Could you check a few things on this model? Use its own coordinates, in mm. Coordinates: 2 decimals unless noted, no trailing zeros. Write each loop counter-clockwise with the first axis right and the second up, starting at its lowest first coordinate (ties: lowest second). Pieces come first, ordered by that corner, then holes. Notation, with made-up numbers: M 22,77 L 80,77 A28 cw 80,112 Z; hole C 49,-13.75 d2. An arc over 180 degrees is marked long. Write item = value, one per line.
```python
from build123d import *

# Parameters (mm, degrees)
ESBO_O1_W                = 14
ESBO_O1_H                = 14
RESSALTO_EXTRUS_O1_DEPTH = 3.175
CORTE_EXTRUS_O1_DEPTH    = 15
ESBO_O10_R               = 1.5
CORTE_EXTRUS_O2_DEPTH    = 4.175


with BuildPart() as part:
    # Esboço1 → Ressalto-extrusão1 (new body)
    with BuildSketch(Plane.XY):
        Rectangle(ESBO_O1_W, ESBO_O1_H)
    extrude(amount=RESSALTO_EXTRUS_O1_DEPTH)

    # Esboço2 → Corte-extrusão1 (cut, through all)
    with BuildSketch(Plane.XZ.offset(7)):
        Polygon((-4, 3.175), (-7, 3.175), (-7, 0), align=None)
        Polygon((4, 3.175), (7, 3.175), (7, 0), align=None)
    extrude(amount=-CORTE_EXTRUS_O1_DEPTH, mode=Mode.SUBTRACT)

    # Esboço10 → Corte-extrusão2 (cut, through all)
    with BuildSketch(Plane.XY.offset(3.175)):
        Circle(ESBO_O10_R)
    extrude(amount=-CORTE_EXTRUS_O2_DEPTH, mode=Mode.SUBTRACT)


solid = part.part
```
Item 1: Imagine slicing it at C-C (z = 2.2). Write out the boundary of the cut face in (x, y), and give its area (3 significant figures).
Numbers:
outline = M -4.92,-7 L 4.92,-7 L 4.92,7 L -4.92,7 Z; hole C 0,0 d3
area = 131 mm²
Item 2: Imagine slicing it at D-D (y = -4.5). Write out the boundary of the cut face in (x, z) (3 decimals), and give its area (3 significant figures).
Numbers:
outline = M -7,0 L 7,0 L 4,3.175 L -4,3.175 Z
area = 34.9 mm²
Item 3: Imagine slicing it at B-B (y = 0). Write out the boundary of the cut face in (x, z) (3 decimals), and give its area (3 significant figures).
Numbers:
outline = M -7,0 L -1.5,0 L -1.5,3.175 L -4,3.175 Z; M 1.5,0 L 7,0 L 4,3.175 L 1.5,3.175 Z
area = 25.4 mm²
Item 4: If we mould it in two halves opening along Y, with no side actions, what happens to faces 1 (the face through (-1.5, 0.07, 1.61)), 2 (the face through (5.521, -0.098, 1.565)), 3 (the face through (0, 7, 2))? For each: pulls with the +Y half, pulls with the -Y half, needs draft (parallel to the pull), parting line crosses it, or undercut.
Numbers:
face_1 = undercut
face_2 = needs draft
face_3 = pulls with the +Y half
Item 5: Imagine slicing it at A-A (x = 0). Write out the boundary of the cut face in (y, z) (3 decimals), and give its area (3 significant figures).
Numbers:
outline = M -7,0 L -1.5,0 L -1.5,3.175 L -7,3.175 Z; M 1.5,0 L 7,0 L 7,3.175 L 1.5,3.175 Z
area = 34.9 mm²
Item 6: If I drill on line 1 along Y through (x, z) = (0, 2.5); line 2 along X through (y, z) = (0.25, 1.1); line 3 along Z through (x, y) = (-5, 1.5), over which ranges is the centre line in solid material (lowest first)?
Numbers:
line_1 = -7 to -1.5, 1.5 to 7
line_2 = -5.96 to -1.48, 1.48 to 5.96
line_3 = 0 to 2.12
